The drawing under review shows one solid part. Ordinate dimensions are in mm from its lowest x, y, z. A direction names the side the tool comes from. Round coordinates to 2 decimals unless told otherwise and drop trailing zeros. Order: outer loops, then holes, each group sorted by start corner. A loop starts at its lowest first (then second) coordinate and runs counter-clockwise, first axis right, second up. Notation, with made-up numbers: M 76,69 L 109,69 A30 ccw 109,98 Z; hole C 37.25,53 d10. An arc over 180 degrees is marked long. Answer as a JSON object with one key per item and string values. Group by question number.
1. To check wall thickness, follow probe 1 along X at (y, z) = (3, 1.45); probe 2 along Z at (x, y) = (7.75, 2.35); probe 3 along Y at (x, z) = (1.5, 1.85). State the ranges of each line that lie inside material, in increasing order. Write a range as [from, to].
2. Clearance check with a flat-ended pin moving along its axis: P1, Ø0.7, axis at y = 2.5, z = 2, coming from the -X side. State where the tip first meets the part, or that it passes through.
3. Add section B-B on y = 2.2. State the section outline as (x, z) points, and give its area (3 significant figures).
4. Add section A-A on z = 1.55. State the section outline as (x, y) points.
5. Add section C-C on x = 7.5. State the section outline as (y, z) points.
6. Add section D-D on y = 1. State the section outline as (x, z) points.
7. Mouldability with a two-part tool opening along X and no side actions: class the marked faces 4, 5 and 6 as released by +X, released by -X, zero draft, split by the parting line, or undercut.
8. Machinability: for the marked faces 1, 2 and 3, which of the approach directions +Z, -Z, +X, -X, +Y, -Y give a long, thin tool a straight path to every point of the face, cutting with its end or side? Answer none if there is none.
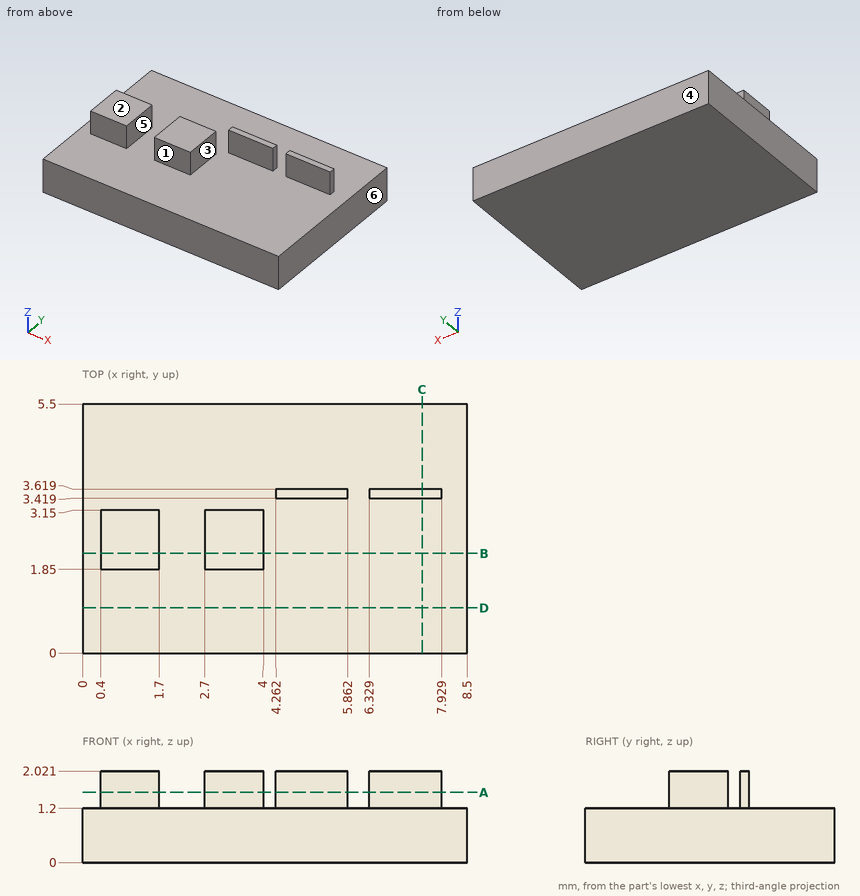
Recorded:
{
 "1": {"probe 1": "x = [0.4, 1.7], [2.7, 4]", "probe 2": "z = [0, 1.2]", "probe 3": "y = [1.85, 3.15]"},
 "2": {"P1": "stops at x = 0.4"},
 "3": {"outline": "M 0,0 L 8.5,0 L 8.5,1.2 L 4,1.2 L 4,2.02 L 2.7,2.02 L 2.7,1.2 L 1.7,1.2 L 1.7,2.02 L 0.4,2.02 L 0.4,1.2 L 0,1.2 Z", "area": "12.3 mm²"},
 "4": {"outline": "M 0.4,1.85 L 1.7,1.85 L 1.7,3.15 L 0.4,3.15 Z; M 2.7,1.85 L 4,1.85 L 4,3.15 L 2.7,3.15 Z; M 4.26,3.42 L 5.86,3.42 L 5.86,3.62 L 4.26,3.62 Z; M 6.33,3.42 L 7.93,3.42 L 7.93,3.62 L 6.33,3.62 Z"},
 "5": {"outline": "M 0,0 L 5.5,0 L 5.5,1.2 L 3.62,1.2 L 3.62,2.02 L 3.42,2.02 L 3.42,1.2 L 0,1.2 Z"},
 "6": {"outline": "M 0,0 L 8.5,0 L 8.5,1.2 L 0,1.2 Z"},
 "7": {"face 4": "zero draft", "face 5": "undercut", "face 6": "released by +X"},
 "8": {"face 1": "+Z, +X, -X, -Y", "face 2": "+Z, +X, -X, +Y, -Y", "face 3": "+Z, +X, +Y, -Y"}
}
